Geometry: see drawing. Coordinates: mm, zero at the bounding-box minimum. A direction names the side the tool comes from. Coordinates: 2 decimals unless noted, no trailing zeros. Write each loop counter-clockwise with the first axis right and the second up, starting at its lowest first coordinate (ties: lowest second). Pieces come first, ordered by that corner, then holes. Notation, with made-up numbers: (89, -17.75) - (123, -17.75) arc R21 cw to (123, -5.75) - close; hole circle Ø4 at (-12.5, 9). An arc over 180 degrees is marked (long way). One line per question, with ' | ' between items. Start each with the question number.
Q1. Cut plane C-C, the plane y = 2.75. Return loops of the section in (x, z), plus the area to 3 significant figures.
Q2. Draft query along X for the marked faces 1, 2 and 3. Return one class per face: +X half, -X half, draft (parallel to the pull), parting line (faces both ways), or undercut.
Q3. Access query for the marked faces 4 and 5. Directions: +Z, -Z, +X, -X, +Y, -Y. A direction counts if a zero-diameter tool reaches every point of the face in a straight line with its end or side. Return the directions, or none.
Q4. Cut plane D-D, the plane y = 16.25. Return loops of the section in (x, z), plus the area to 3 significant figures.
Q5. Contact query for flat-ended pins moving along their axis: P1, Ø5, axis at x = 7, z = 15, coming from the -Y side; P2, Ø11, axis at x = 67, z = 15, coming from the -Y side. Output: stop coordinate, or through.
Q6. Cut plane B-B, the plane z = 15. Return loops of the section in (x, y).
Q7. Cut plane A-A, the plane x = 10.5. Return loops of the section in (y, z), plus the area to 3 significant figures.
Q8. Line query: line 1 (X direction, y = 21.5, z = 15); line 2 (Y direction, x = 17, z = 23); line 3 (Z direction, x = 67, y = 15.25). Output: solid intervals per line, ascending.
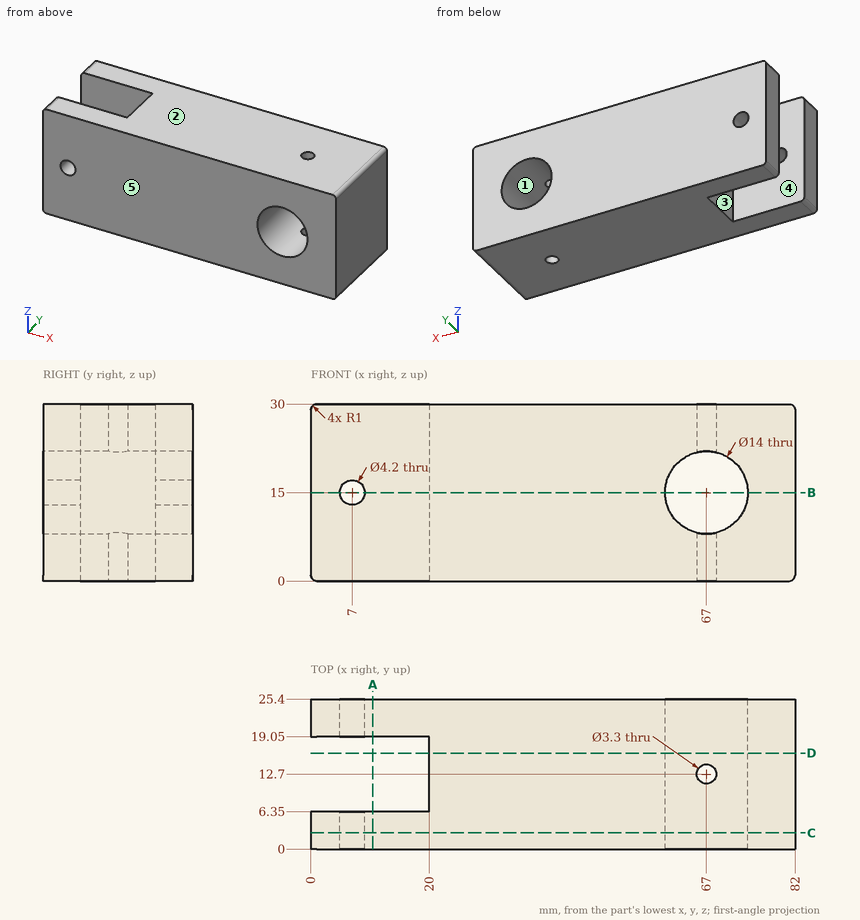
Reply:
1) outline: (0, 1) arc R1 ccw to (1, 0) - (81, 0) arc R1 ccw to (82, 1) - (82, 29) arc R1 ccw to (81, 30) - (1, 30) arc R1 ccw to (0, 29) - close; hole circle Ø4.2 at (7, 15); hole circle Ø14 at (67, 15) | area: 2,290 mm^2
2) face 1: undercut | face 2: draft | face 3: -X half
3) face 4: +Z, -Z, -X | face 5: +Z, -Z, +X, -X, -Y
4) outline: (20, 0) - (81, 0) arc R1 ccw to (82, 1) - (82, 29) arc R1 ccw to (81, 30) - (20, 30) - close; hole circle Ø14 at (67, 15) | area: 1,710 mm^2
5) P1: stops at y = 0 | P2: passes through
6) outline: (0, 0) - (4.9, 0) - (4.9, 6.35) - (0, 6.35) - close; (0, 19.05) - (4.9, 19.05) - (4.9, 25.4) - (0, 25.4) - close; (9.1, 0) - (60, 0) - (60, 25.4) - (9.1, 25.4) - (9.1, 19.05) - (20, 19.05) - (20, 6.35) - (9.1, 6.35) - close; (74, 0) - (82, 0) - (82, 25.4) - (74, 25.4) - close
7) outline: (0, 0) - (6.35, 0) - (6.35, 30) - (0, 30) - close; (19.05, 0) - (25.4, 0) - (25.4, 30) - (19.05, 30) - close | area: 381 mm^2
8) line 1: x = 0 to 4.9, 9.1 to 60, 74 to 82 | line 2: y = 0 to 6.35, 19.05 to 25.4 | line 3: z = 0 to 8, 22 to 30
